```python
from build123d import *

# Parameters (mm, degrees)
SKETCH1_W           = 508
SKETCH1_H           = 25.4
BOSS_EXTRUDE1_DEPTH = 12.7
SKETCH3_R           = 9.525
BOSS_EXTRUDE2_DEPTH = 76.2
SWEEP1_PROFILE_R    = 9.525


with BuildPart() as part:
    # Sketch1 → Boss-Extrude1 (new body)
    with BuildSketch(Plane(origin=(0, 0, 0), x_dir=(1, 0, 0), z_dir=(0, 1, 0))):
        Rectangle(SKETCH1_W, SKETCH1_H)
    extrude(amount=BOSS_EXTRUDE1_DEPTH)

    # Sketch3 → Boss-Extrude2 (add)
    with BuildSketch(Plane.XZ):
        with Locations(Location((-127, 0, 0), (0, 0, 90))):
            Circle(SKETCH3_R)
        with Locations(Location((127, 0, 0), (0, 0, 90))):
            Circle(SKETCH3_R)
    extrude(amount=BOSS_EXTRUDE2_DEPTH)

    # Sweep1: sweep along a path in Sketch4
    with BuildLine(Plane.XY) as sweep1_path:
        Line((-228.6, 12.7), (-228.6, 152.4))
        ThreePointArc((-228.6, 152.4), (-232.319743879, 161.380256121), (-241.3, 165.1))
        Line((-241.3, 165.1), (-279.4, 165.1))
    # Sweep1 profile (on start of the path) → Sweep1 (sweep)
    with BuildSketch(Plane(origin=(-228.6, 12.7, 0), x_dir=(0, 0, 1), z_dir=(0, 1, 0))):
        Circle(SWEEP1_PROFILE_R)
    sweep1 = sweep(path=sweep1_path.line)

    # Mirror1: Sweep1 across plane
    add(sweep1.mirror(Plane(origin=(0, 0, 0), x_dir=(0, 0, 1), z_dir=(1, 0, 0))))


solid = part.part
```
Build history of the part. All positions in model axes, mm. A direction names the side the tool comes from. Round coordinates to 2 decimals unless told otherwise and drop trailing zeros. Write each loop counter-clockwise with the first axis right and the second up, starting at its lowest first coordinate (ties: lowest second). Pieces come first, ordered by that corner, then holes.
1) Band-saw the part on A-A, the plane y = 44. List the corners of the cut face in (x, z) (3 decimals), and give its area (3 significant figures).
2) Band-saw the part on B-B, the plane x = -127. List the corners of the cut face in (y, z) (3 decimals).
3) 3-axis set-ups, long thin cutter, end or side, ignore diameter. For faces 1 (the cylindrical face through (-136.444, -37.567, -1.24)), 2 (the cylindrical face through (-260.617, 174.544, -1.24)), 3 (the cylindrical face through (260.617, 174.544, -1.24)), 4 (the cylindrical face through (237.9, 83.53, -2.06)): which of +Z, -Z, +X, -X, +Y, -Y reach the whole face in a straight line?
4) Drill centre lines: probe 1 along Y at (x, z) = (102, -1); probe 2 along X at (y, z) = (79, -5.5); probe 3 along X at (y, z) = (112.5, 0.5). Where is each one in solid material? Low to high.
5) Band-saw the part on C-C, the plane z = 3.5. List the corners of the cut face in (x, y).
6) Pin check, flat tips, straight feed: pin 1 (8 mm diameter, centred on y = 38.5, z = 0.5, fed in from -X) (3 decimals); pin 2 (8 mm diameter, centred on y = -5, z = -3.5, fed in from +X) (3 decimals); pin 3 (4 mm diameter, centred on y = -26, z = -9, fed in from -X). Stop position of each tip, or through.
7) Mould opens along X. For faces 5 (the flat face through (-254, 6, 0)), 6 (the cylindrical face through (117.556, -37.567, -1.24)), 7 (the flat face through (-4, 6, 12.7)) say: +X half, -X half, draft (parallel to the pull), parting line (faces both ways), or undercut.
8) Band-saw the part on D-D, the plane x = -49.5. List the corners of the cut face in (y, z).
Ans:
1. outline: circle Ø19.05 at (-228.6, 0); circle Ø19.05 at (228.6, 0)
1. area: 570 mm2
2. outline: (-76.2, -9.525) - (0, -9.525) - (0, -12.7) - (12.7, -12.7) - (12.7, 12.7) - (0, 12.7) - (0, 9.525) - (-76.2, 9.525) - close
3. face 1: -Y
3. face 2: -X
3. face 3: +X
3. face 4: none
4. probe 1: y = 0 to 12.7
4. probe 2: x = -236.38 to -220.82, 220.82 to 236.38
4. probe 3: x = -238.11 to -219.09, 219.09 to 238.11
5. outline: (-279.4, 156.24) - (-241.3, 156.24) arc R3.84 cw to (-237.46, 152.4) - (-237.46, 12.7) - (-254, 12.7) - (-254, 0) - (-135.86, 0) - (-135.86, -76.2) - (-118.14, -76.2) - (-118.14, 0) - (118.14, 0) - (118.14, -76.2) - (135.86, -76.2) - (135.86, 0) - (254, 0) - (254, 12.7) - (237.46, 12.7) - (237.46, 152.4) arc R3.84 cw to (241.3, 156.24) - (279.4, 156.24) - (279.4, 173.96) - (241.3, 173.96) arc R21.56 ccw to (219.74, 152.4) - (219.74, 12.7) - (-219.74, 12.7) - (-219.74, 152.4) arc R21.56 ccw to (-241.3, 173.96) - (-279.4, 173.96) - close
6. pin 1: stops at x = -238.125
6. pin 2: stops at x = 136.525
6. pin 3: stops at x = -133.46
7. face 5: -X half
7. face 6: undercut
7. face 7: draft
8. outline: (0, -12.7) - (12.7, -12.7) - (12.7, 12.7) - (0, 12.7) - close
